```python
from build123d import *

# Parameters (mm, degrees)
SKETCH1_W           = 76.2
SKETCH1_H           = 50.8
BOSS_EXTRUDE1_DEPTH = 6.35
SKETCH2_W           = 12.7
SKETCH2_H           = 3.175
BOSS_EXTRUDE2_DEPTH = 10.16
FILLET1_R           = 2.54
CUT_EXTRUDE1_REACH  = 63.293
SKETCH3_R           = 1.5875


with BuildPart() as part:
    # Sketch1 → Boss-Extrude1 (new body)
    with BuildSketch(Plane(origin=(0, 0, 0), x_dir=(0, 0, -1), z_dir=(1, 0, 0))):
        Rectangle(SKETCH1_W, SKETCH1_H)
    extrude(amount=BOSS_EXTRUDE1_DEPTH)

    # Sketch2 → Boss-Extrude2 (add)
    with BuildSketch(Plane(origin=(6.35, 0, 0), x_dir=(0, 0, -1), z_dir=(1, 0, 0))):
        with Locations((0, -18.0975)):
            Rectangle(SKETCH2_W, SKETCH2_H)
        with Locations((0, 18.0975)):
            Rectangle(SKETCH2_W, SKETCH2_H)
    extrude(amount=BOSS_EXTRUDE2_DEPTH)

    # Fillet1
    fillet1_edges = [part.edges().sort_by_distance(p)[0] for p in [
        (0, 25.4, 0),
        (0, 0, -38.1),
        (0, -25.4, 0),
        (0, 0, 38.1),
        (3.175, 25.4, 38.1),
        (3.175, 25.4, -38.1),
        (3.175, -25.4, -38.1),
        (3.175, -25.4, 38.1),
    ]]
    fillet(fillet1_edges, radius=FILLET1_R)

    # Cut-Extrude1: up to this face of the body (flat: up to its plane)
    cut_extrude1_end = Plane(part.part.faces().sort_by_distance((11.43, -19.685, 0))[0])
    # Sketch3 → Cut-Extrude1 (cut, up to the picked face)
    with BuildSketch(Plane(origin=(0, 19.685, 0), x_dir=(1, 0, 0), z_dir=(0, 1, 0)), mode=Mode.PRIVATE) as cut_extrude1_sk1:
        with Locations(Location((11.43, -3.175, 0), (0, 0, 270))):
            Circle(SKETCH3_R)
    cut_extrude1_tool1 = split(extrude(cut_extrude1_sk1.sketch, amount=-CUT_EXTRUDE1_REACH, mode=Mode.PRIVATE), bisect_by=cut_extrude1_end, keep=Keep.BOTH, mode=Mode.PRIVATE)
    # Sketch3 → Cut-Extrude1 (cut, up to the picked face)
    with BuildSketch(Plane(origin=(0, 19.685, 0), x_dir=(1, 0, 0), z_dir=(0, 1, 0)), mode=Mode.PRIVATE) as cut_extrude1_sk2:
        with Locations(Location((11.43, 3.175, 0), (0, 0, 270))):
            Circle(SKETCH3_R)
    cut_extrude1_tool2 = split(extrude(cut_extrude1_sk2.sketch, amount=-CUT_EXTRUDE1_REACH, mode=Mode.PRIVATE), bisect_by=cut_extrude1_end, keep=Keep.BOTH, mode=Mode.PRIVATE)
    add(cut_extrude1_tool1.solids().sort_by(Axis((11.43, 19.685, 3.175), (0, -1, 0)))[0], mode=Mode.SUBTRACT)
    add(cut_extrude1_tool2.solids().sort_by(Axis((11.43, 19.685, -3.175), (0, -1, 0)))[0], mode=Mode.SUBTRACT)


solid = part.part
```
Verification items for the finished model (mm, model axes). A direction names the side the tool comes from. Give positions to 0.01 mm unless a question says otherwise; leave off trailing zeros. Order: outer loops, then holes, each group sorted by start corner. A loop starts at its lowest first (then second) coordinate and runs counter-clockwise, first axis right, second up. Notation, with made-up numbers: M 30.5,20.25 L 38.5,20.25 A28 cw 38.5,47.25 Z; hole C 66.5,-10.5 d9. An arc over 180 degrees is marked long. Answer in a Markdown table with one row per item. Add a question column.
Item 1: Tool access check on faces 4 (the flat face through (11, -19.685, 0)), 5 (the flat face through (11, -18, -6.35)), 6 (the flat face through (11, 16.51, 0)). Record the directions out of +Z, -Z, +X, -X, +Y, -Y that give a thin tool (end or side, any length) a straight path to the whole face; none if there is none.
Item 2: Section check A-A, the plane x = 11.43. State how many separate pieces and enclosed holes the cut face has, and give its area (3 significant figures).
Item 3: Section check C-C, the plane y = -10. Enter the section's corners in (x, z), and give its area (3 significant figures).
Item 4: Scan lines: probe 1 along Y at (x, z) = (16.25, 0) (3 decimals); probe 2 along X at (y, z) = (17.5, -14.5); probe 3 along Z at (x, y) = (12.75, -18). Record each from-to range of solid material in increasing order. Write a range as from..to.
Item 5: Gauge pin test, flat ends, axial feed: pin 1 (3 mm diameter, centred on x = 12.5, z = 3, fed in from +Y) (3 decimals); pin 2 (1 mm diameter, centred on x = 12.5, y = 17.5, fed in from -Z); pin 3 (4 mm diameter, centred on x = 11.43, z = -3.175, fed in from -Y) (3 decimals); pin 4 (2 mm diameter, centred on x = 12.5, z = -8.5, fed in from +Y). Record the tip position at first contact, or that the pin passes through.
Item 6: Mould release check, pull along Z, two halves, no side actions. Record for faces 1 (the cylindrical face through (4.472, -24.636, 37.376)), 2 (the cylindrical face through (11.91, 18.12, -1.66)), 3 (the flat face through (0, 0, 0)): released by +Z, released by -Z, zero draft, split by the parting line, or undercut.
Item 7: Section check B-B, the plane z = -8.5. Enter the section's corners in (x, y), and give its area (3 significant figures).
Filled sheet:
| question | item | result |
|---|---|---|
| 1 | face 4 | +Z, -Z, +X, -Y |
| 1 | face 5 | -Z, +X, +Y, -Y |
| 1 | face 6 | +Z, -Z, +X |
| 2 | separate pieces | 6 |
| 2 | enclosed holes | 0 |
| 2 | area | 40.3 mm^2 |
| 3 | outline | M 0,-35.56 A2.54 ccw 2.54,-38.1 L 6.35,-38.1 L 6.35,38.1 L 2.54,38.1 A2.54 ccw 0,35.56 Z |
| 3 | area | 481 mm^2 |
| 4 | probe 1 | y = -19.685..-16.51, 16.51..19.685 |
| 4 | probe 2 | x = 0..6.35 |
| 4 | probe 3 | z = -6.35..-4.06, -2.29..2.29, 4.06..6.35 |
| 5 | pin 1 | stops at y = 19.685 |
| 5 | pin 2 | stops at z = -6.35 |
| 5 | pin 3 | stops at y = -19.685 |
| 5 | pin 4 | passes through |
| 6 | face 1 | released by +Z |
| 6 | face 2 | undercut |
| 6 | face 3 | zero draft |
| 7 | outline | M 0,-22.86 A2.54 ccw 2.54,-25.4 L 6.35,-25.4 L 6.35,25.4 L 2.54,25.4 A2.54 ccw 0,22.86 Z |
| 7 | area | 320 mm^2 |
